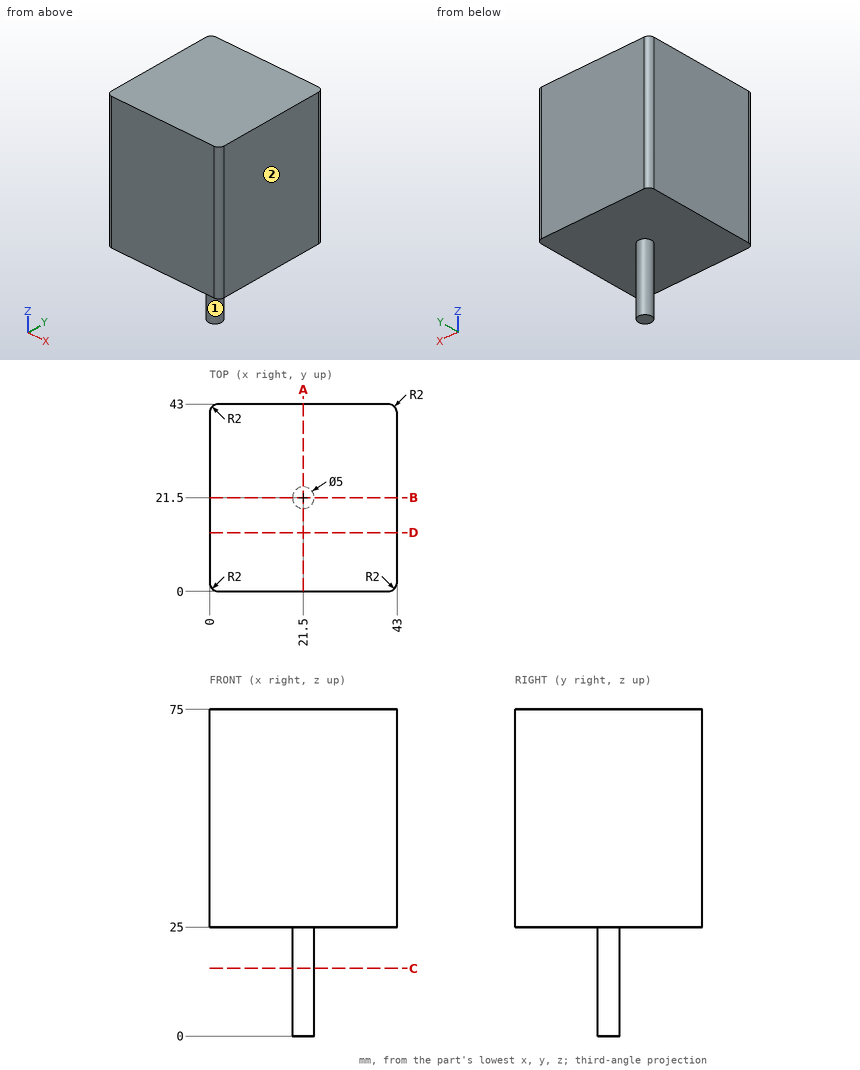
Could you check a few things on this drawing? It's one solid part, dimensions in mm from its lowest x, y, z. A direction names the side the tool comes from. Round coordinates to 2 decimals unless told otherwise and drop trailing zeros. Order: outer loops, then holes, each group sorted by start corner. A loop starts at its lowest first (then second) coordinate and runs counter-clockwise, first axis right, second up. Notation, with made-up numbers: M 27.5,62 L 32.5,62 A31 ccw 32.5,87 Z; hole C 71,21 d3. An arc over 180 degrees is marked long. One line per question, with ' | ' between items.
1) Imagine slicing it at C-C, the plane z = 15.5. Write out the boundary of the cut face in (x, y), plus the area to 3 significant figures.
Checked values:
outline: C 21.5,21.5 d5 | area: 19.6 mm²
2) Imagine slicing it at D-D, the plane y = 13.5. Write out the boundary of the cut face in (x, z), plus the area to 3 significant figures.
Checked values:
outline: M 0,25 L 43,25 L 43,75 L 0,75 Z | area: 2,150 mm²
3) I'm going to push flat-ended pins straight in: pin 1 Ø13 at (x, y) = (24.5, 23.5) entering from -Z; pin 2 Ø3 at (x, y) = (5, 35) entering from -Z; pin 3 Ø10 at (x, z) = (21.5, 11) entering from +Y. Where does each tip first touch, or does it pass through?
Checked values:
pin 1: stops at z = 0 | pin 2: stops at z = 25 | pin 3: stops at y = 24
4) Imagine slicing it at A-A, the plane x = 21.5. Write out the boundary of the cut face in (y, z).
Checked values:
outline: M 0,25 L 19,25 L 19,0 L 24,0 L 24,25 L 43,25 L 43,75 L 0,75 Z
5) I need wall thicknesses on line 1 (Z direction, x = 10.5, y = 14); line 2 (X direction, y = 19.5, z = 10.5); line 3 (X direction, y = 41.5, z = 40). Which ranges of each line are inside material? Lowest first, please.
Checked values:
line 1: z = 25 to 75 | line 2: x = 20 to 23 | line 3: x = 0.06 to 42.94
6) On a 3-axis mill with a long thin cutter (end or side, diameter ignored), from which of +Z, -Z, +X, -X, +Y, -Y can I reach the whole of each face in a straight line? I mean the marked faces 1 and 2. Say none if no direction works.
Checked values:
face 1: -Z | face 2: +Z, -Z, +X, +Y, -Y
